from build123d import *

# Parameters (mm, degrees)
F0_W     = 152.3603492588
F0_H     = 50.8
F1_DEPTH = 101.6
F2_W     = 152.4
F2_H     = 50.8
F3_DEPTH = 25.4
F4_W     = 50.8
F4_H     = 50.8
F5_DEPTH = 76.2


with BuildPart() as f1:
    # F0 (on Front) → F1 (new body)
    with BuildSketch(Plane.XZ):
        Polygon((-47.2552540332, -18.1309473828), (-98.0552540332, -18.1309473828), (-98.0552540332, -119.7309473828), (-47.215603292, -119.7309473828), (-47.215603292, -68.9309473828), (-47.2552540332, -68.9309473828), align=None)
        with Locations((28.9645713374, -94.3309473828)):
            Rectangle(F0_W, F0_H)
    extrude(amount=-F1_DEPTH)

    # F2 (on Front) → F3 (cut)
    with BuildSketch(Plane.XZ):
        with Locations((28.9447459668, -94.3309473828)):
            Rectangle(F2_W, F2_H)
    extrude(amount=-F3_DEPTH, mode=Mode.SUBTRACT)

    # F4 (on Front) → F5 (cut)
    with BuildSketch(Plane.XZ):
        with Locations((-72.6552540332, -43.0878863094)):
            Rectangle(F4_W, F4_H)
    extrude(amount=-F5_DEPTH, mode=Mode.SUBTRACT)


solid = f1.part
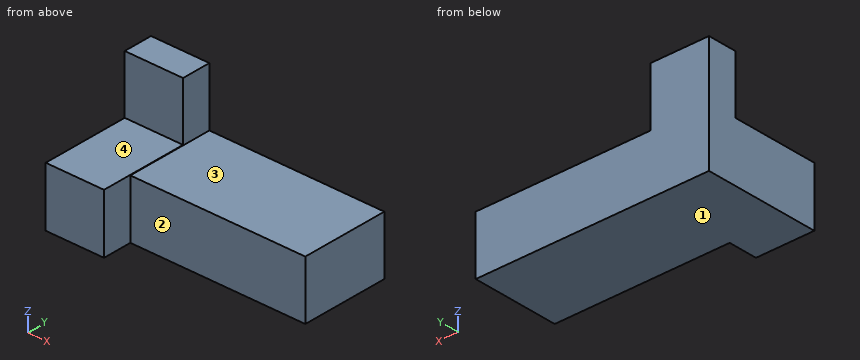
Can you work these out from the model? Positions are in its coordinate system, mm. Face numbers are marked on the shaded views. A direction names the side the tool comes from. Coordinates: 2 decimals unless noted, no trailing zeros. Write each loop counter-clockwise with the first axis right and the second up, starting at its lowest first coordinate (ties: lowest second). Pieces come first, ordered by that corner, then holes. Notation, with made-up numbers: (39, 43.5) -> (61, 43.5) arc R23 ccw to (61, 63.5) -> close; hole circle Ø10 at (9, 57.5). An arc over 180 degrees is marked (long way). Write each question's results on one line, items separated by ' | '. Start each with the question number.
Item 1: If we section it at B-B, the plane z = -87.5: Write out the boundary of the cut face in (x, y), and give its area (3 significant figures).
Item 2: On a 3-axis mill with a long thin cutter (end or side, diameter ignored), from which of +Z, -Z, +X, -X, +Y, -Y can I reach the whole of each face in a straight line? I mean the marked faces 1, 2, 3 and 4. Say none if no direction works.
Item 3: If we section it at D-D, the plane z = -31: Write out the boundary of the cut face in (x, y).
Item 4: Please list where these lines run through material, in increasing order: probe 1 along Z at (x, y) = (55.5, 53); probe 2 along Y at (x, z) = (30, -110.5); probe 3 along X at (y, z) = (17, -89).
Item 5: If we section it at C-C, the plane x = 63: Write out the boundary of the cut face in (y, z), and give its area (3 significant figures).
Item 6: I'm going to push flat-ended pins straight in: P1, Ø1.5, axis at x = -45, y = 86, coming from the +Z side; P2, Ø6, axis at x = 7, z = -101.5, coming from the -Y side; P3, Ø15, axis at x = -65, z = -39.5, coming from the -Y side. Where does each tip first touch, or does it pass through?
Item 7: If we section it at A-A, the plane y = 94.5: Write out the boundary of the cut face in (x, z).
Answer block:
1) outline: (-98.06, 0) -> (-47.26, 0) -> (-47.26, 25.4) -> (105.14, 25.4) -> (105.14, 101.6) -> (-98.06, 101.6) -> close | area: 16,800 mm²
2) face 1: -Z, +X, -X, +Y, -Y | face 2: +Z, -Z, +X, -Y | face 3: +Z, +X, +Y, -Y | face 4: +Z, +X, -X, -Y
3) outline: (-98.06, 76.2) -> (-47.26, 76.2) -> (-47.26, 101.6) -> (-98.06, 101.6) -> close
4) probe 1: -119.73 to -68.93 | probe 2: 25.4 to 101.6 | probe 3: -98.06 to -47.26
5) outline: (25.4, -119.73) -> (101.6, -119.73) -> (101.6, -68.93) -> (25.4, -68.93) -> close | area: 3,870 mm²
6) P1: z = -68.93 | P2: y = 25.4 | P3: y = 76.2
7) outline: (-98.06, -119.73) -> (105.14, -119.73) -> (105.14, -68.93) -> (-47.26, -68.93) -> (-47.26, -18.13) -> (-98.06, -18.13) -> close
